CAD build for the part. Positions are in the model's coordinates, mm. A direction names the side the tool comes from. Give positions to 0.01 mm unless a question says otherwise; leave off trailing zeros. Answer as a JSON object with one key per item and string values.
```python
from build123d import *

# Parameters (mm, degrees)
CROQUIS1_R                          = 33
CROQUIS1_R_2                        = 29
BOSS_EXTRUDE1_DEPTH                 = 92
BOSS_EXTRUDE4_DEPTH                 = 15
SKETCH9_R                           = 1.75
CUT_EXTRUDE3_DEPTH                  = 14
SKETCH10_W                          = 7
SKETCH10_H                          = 15
SKETCH10_W_2                        = 8
SKETCH10_H_2                        = 13
CORTE_USB_Y_SWITCH_DEPTH            = 10
SKETCH11_W                          = 8
SKETCH11_H                          = 13
CUT_EXTRUDE5_DEPTH                  = 10
ALOJAMIENTO_TUERCA_DEPTH            = 2.2
ALOJAMIENTOS_TUERCAS_SUPERIOR_COUNT = 4
GROSOR_START                        = -47
SKETCH13_R                          = 29
SKETCH13_R_2                        = 26
GROSOR_ADICIONAL_DEPTH              = 47
CORTE_REVOLUCION_W                  = 30
CORTE_REVOLUCION_H                  = 8
CUT_REVOLVE3_ANGLE                  = 57
CIRPATTERN3_COUNT                   = 3
CORTE_POSTIZOS_DEPTH                = 44
CHAMFER3_SIZE                       = 3
SKETCH14_R                          = 1.75
CUT_EXTRUDE6_DEPTH                  = 17
TUERCAS_INFERIOR_DEPTH              = 2.2


with BuildPart() as part:
    # Croquis1 → Boss-Extrude1 (new body)
    with BuildSketch(Plane.XY):
        Circle(CROQUIS1_R)
        Circle(CROQUIS1_R_2, mode=Mode.SUBTRACT)
    extrude(amount=BOSS_EXTRUDE1_DEPTH)

    # Sketch8 → Boss-Extrude4 (add)
    with BuildSketch(Plane(origin=(0, 0, 0), x_dir=(-1, 0, 0), z_dir=(0, 0, -1))):
        with BuildLine():
            ThreePointArc((-4, -28.722813233), (0, -29), (4, -28.722813233))
            ThreePointArc((4, -28.722813233), (0, -26.000786616), (-4, -28.722813233))
        make_face()
        with BuildLine():
            ThreePointArc((-28.722813233, 4), (-29, 0), (-28.722813233, -4))
            ThreePointArc((-28.722813233, -4), (-26.000786616, 0), (-28.722813233, 4))
        make_face()
        with BuildLine():
            ThreePointArc((4, 28.722813233), (0, 29), (-4, 28.722813233))
            ThreePointArc((-4, 28.722813233), (0, 26.000786616), (4, 28.722813233))
        make_face()
        with BuildLine():
            ThreePointArc((28.722813233, -4), (29, 0), (28.722813233, 4))
            ThreePointArc((28.722813233, 4), (26.000786616, 0), (28.722813233, -4))
        make_face()
    extrude(amount=-BOSS_EXTRUDE4_DEPTH)

    # Sketch9 → Cut-Extrude3 (cut)
    with BuildSketch(Plane(origin=(0, 0, 0), x_dir=(-1, 0, 0), z_dir=(0, 0, -1))):
        with Locations((0, -29)):
            Circle(SKETCH9_R)
        with Locations((-29, 0)):
            Circle(SKETCH9_R)
        with Locations((0, 29)):
            Circle(SKETCH9_R)
        with Locations((29, 0)):
            Circle(SKETCH9_R)
    extrude(amount=-CUT_EXTRUDE3_DEPTH, mode=Mode.SUBTRACT)

    # Sketch10 → Corte USB y Switch (cut)
    with BuildSketch(Plane(origin=(-23.334523779, -23.334523779, 0), x_dir=(0, 0, -1), z_dir=(-0.7071067811865488, -0.7071067811865464, 0))):
        with Locations((-7, 0)):
            Rectangle(SKETCH10_W, SKETCH10_H)
        with Locations((-38, 0)):
            Rectangle(SKETCH10_W_2, SKETCH10_H_2)
    extrude(amount=-CORTE_USB_Y_SWITCH_DEPTH, mode=Mode.SUBTRACT)

    # Sketch11 → Cut-Extrude5 (cut)
    with BuildSketch(Plane(origin=(12.362017583, 30.597067201, 0), x_dir=(0, 0, -1), z_dir=(0.37460659341590646, 0.9271838545667896, 0))):
        with Locations((-26.9, -0.5)):
            Rectangle(SKETCH11_W, SKETCH11_H)
    extrude(amount=-CUT_EXTRUDE5_DEPTH, mode=Mode.SUBTRACT)

    # Tuerca → Alojamiento tuerca (cut)
    with BuildSketch(Plane(origin=(0, 0, 3), x_dir=(-1, 0, 0), z_dir=(0, 0, -1))):
        with BuildLine():
            Line((-29, -3.406366588), (-25.579878574, -3.406366588))
            ThreePointArc((-25.579878574, -3.406366588), (-23.904124497, 0), (-25.579878574, 3.406366588))
            Line((-25.579878574, 3.406366588), (-29, 3.406366588))
            Line((-29, 3.406366588), (-31.95, 1.703183294))
            Line((-31.95, 1.703183294), (-31.95, -1.703183294))
            Line((-31.95, -1.703183294), (-29, -3.406366588))
        make_face()
    alojamiento_tuerca = extrude(amount=-ALOJAMIENTO_TUERCA_DEPTH, mode=Mode.SUBTRACT)

    # Alojamientos Tuercas Superior: Alojamiento tuerca ×4 about axis
    alojamientos_tuercas_superior_axis = Axis((0, 0, 0), (0, 0, 1))
    for i in range(1, ALOJAMIENTOS_TUERCAS_SUPERIOR_COUNT):
        add(alojamiento_tuerca.rotate(alojamientos_tuercas_superior_axis, i * 360 / ALOJAMIENTOS_TUERCAS_SUPERIOR_COUNT), mode=Mode.SUBTRACT)

    # Sketch13 → Grosor adicional (add)
    with BuildSketch(Plane.XY.offset(92).offset(GROSOR_START)):
        with Locations(Location((0, 0, 0), (0, 0, 187.928141766))):
            Circle(SKETCH13_R)
        Circle(SKETCH13_R_2, mode=Mode.SUBTRACT)
    extrude(amount=GROSOR_ADICIONAL_DEPTH)

    # Corte Revolucion → Cut-Revolve3 (revolve, cut)
    with BuildSketch(Plane(origin=(0, 0, 0), x_dir=(0, 0, -1), z_dir=(0.2756373558169964, -0.9612616959383197, 0))):
        with Locations((-65, 29)):
            Rectangle(CORTE_REVOLUCION_W, CORTE_REVOLUCION_H)
    cut_revolve3 = revolve(axis=Axis((0, 0, 92), (0, 0, -1)), revolution_arc=CUT_REVOLVE3_ANGLE, mode=Mode.SUBTRACT)

    # CirPattern3: Cut-Revolve3 ×3 about axis
    cirpattern3_axis = Axis((0, 0, 0), (0, 0, 1))
    for i in range(1, CIRPATTERN3_COUNT):
        add(cut_revolve3.rotate(cirpattern3_axis, i * 360 / CIRPATTERN3_COUNT), mode=Mode.SUBTRACT)

    # Croquis2 → Corte postizos (cut)
    with BuildSketch(Plane.XY.offset(92)):
        with BuildLine():
            Line((7.72153797, 29.247911915), (7.338651789, 27.797602233))
            ThreePointArc((7.338651789, 27.797602233), (-8.645291736, 27.419362334), (-21.955521244, 18.561184955))
            Line((-21.955521244, 18.561184955), (-23.1010267, 19.529594604))
            ThreePointArc((-23.1010267, 19.529594604), (-9.096350435, 28.84993776), (7.72153797, 29.247911915))
        make_face()
        with BuildLine():
            Line((21.468665741, -21.311003996), (20.404103804, -20.254259996))
            ThreePointArc((20.404103804, -20.254259996), (28.068510205, -6.222638901), (27.052218317, 9.733446673))
            Line((27.052218317, 9.733446673), (28.463638403, 10.241278673))
            ThreePointArc((28.463638403, 10.241278673), (29.532954215, -6.547298322), (21.468665741, -21.311003996))
        make_face()
        with BuildLine():
            Line((-29.190203711, -7.936907919), (-27.742755593, -7.543342237))
            ThreePointArc((-27.742755593, -7.543342237), (-19.423218469, -21.196723433), (-5.096697073, -28.294631628))
            Line((-5.096697073, -28.294631628), (-5.362611703, -29.770873278))
            ThreePointArc((-5.362611703, -29.770873278), (-20.43660378, -22.302639439), (-29.190203711, -7.936907919))
        make_face()
    extrude(amount=-CORTE_POSTIZOS_DEPTH, mode=Mode.SUBTRACT)

    # Chamfer3
    chamfer3_edges = [part.edges().sort_by_distance(p)[0] for p in [
        (-29, 0, 45),
    ]]
    chamfer(chamfer3_edges, length=CHAMFER3_SIZE - 0.0001)  # a hair under: the kernel refuses the full size

    # Sketch14 → Cut-Extrude6 (cut)
    with BuildSketch(Plane.XY.offset(92)):
        with Locations((19.929911125, 21.749681436)):
            Circle(SKETCH14_R)
        with Locations((8.870821085, -28.134650047)):
            Circle(SKETCH14_R)
        with Locations((-28.80073221, 6.384968611)):
            Circle(SKETCH14_R)
    extrude(amount=-CUT_EXTRUDE6_DEPTH, mode=Mode.SUBTRACT)

    # Sketch15 → Tuercas inferior (cut)
    with BuildSketch(Plane.XY.offset(89)):
        with BuildLine():
            Line((17.415459305, 24.047694791), (15.108166619, 21.523089667))
            ThreePointArc((15.108166619, 21.523089667), (16.492116143, 17.98809762), (20.137070258, 16.927062957))
            Line((20.137070258, 16.927062957), (22.444362944, 19.451668081))
            Line((22.444362944, 19.451668081), (23.177274978, 22.778253911))
            Line((23.177274978, 22.778253911), (20.662823159, 25.076267266))
            Line((20.662823159, 25.076267266), (17.415459305, 24.047694791))
        make_face()
        with BuildLine():
            Line((12.118184939, -27.106077572), (11.08545911, -23.84560093))
            ThreePointArc((11.08545911, -23.84560093), (7.332091433, -23.276640352), (4.590731403, -25.90274588))
            Line((4.590731403, -25.90274588), (5.623457232, -29.163222522))
            Line((5.623457232, -29.163222522), (8.137909051, -31.461235877))
            Line((8.137909051, -31.461235877), (11.385272905, -30.432663402))
            Line((11.385272905, -30.432663402), (12.118184939, -27.106077572))
        make_face()
        with BuildLine():
            Line((-29.533644244, 3.058382781), (-26.193625729, 2.322511264))
            ThreePointArc((-26.193625729, 2.322511264), (-23.824207576, 5.288542732), (-24.727801661, 8.975682923))
            Line((-24.727801661, 8.975682923), (-28.067820176, 9.711554441))
            Line((-28.067820176, 9.711554441), (-31.31518403, 8.682981966))
            Line((-31.31518403, 8.682981966), (-32.048096064, 5.356396136))
            Line((-32.048096064, 5.356396136), (-29.533644244, 3.058382781))
        make_face()
    extrude(amount=-TUERCAS_INFERIOR_DEPTH, mode=Mode.SUBTRACT)


solid = part.part
```
1) Slice it at A-A (x = 0). State how many separate pieces and enclosed holes the cut face has, then the cut area to 3 significant figures.
Model answer:
{"separate pieces": "6", "enclosed holes": "0", "area": "777 mm2"}
2) Mould opens along Z. For faces 4 (the conical face through (-20.782, 15.935, 44.812)), 5 (the cylindrical face through (8.491, -29.843, 90.521)), 6 (the flat face through (-20, -23, 80)), 7 (the flat face through (0, 27, 0)) say: released by +Z, released by -Z, zero draft, split by the parting line, or undercut.
Model answer:
{"face 4": "undercut", "face 5": "zero draft", "face 6": "undercut", "face 7": "released by -Z"}
3) Wall check: probe 1 along Y at (x, z) = (0, 8); probe 2 along Z at (x, y) = (25, -18); probe 3 along Y at (x, z) = (-11.5, 87.5). Give the ranges that are in metal, low to high.
Model answer:
{"probe 1": "y = -33 to -30.75, -27.25 to -26, 26 to 27.25, 30.75 to 33", "probe 2": "z = 0 to 50, 80 to 92", "probe 3": "y = -30.93 to -27.98, -26.35 to -23.32, 23.32 to 26.35, 27.98 to 30.93"}
4) Pin check, flat tips, straight feed: pin 1 (3 mm diameter, centred on x = 22.5, z = 39, fed in from +Y); pin 2 (0.7 mm diameter, centred on x = 0.5, z = 4, fed in from -Y); pin 3 (4 mm diameter, centred on y = 4.5, z = 63, fed in from +X). Stop position of each tip, or through.
Model answer:
{"pin 1": "stops at y = 25.46", "pin 2": "stops at y = -33", "pin 3": "stops at x = -25.17"}
5) 3-axis set-ups, long thin cutter, end or side, ignore diameter. For faces 1 (the cylindrical face through (-12.845, 27.387, 84.975)), 2 (the flat face through (-26.047, -16.855, 38.056)), 3 (the flat face through (7, -27, 86.8)): which of +Z, -Z, +X, -X, +Y, -Y reach the whole face in a straight line?
Model answer:
{"face 1": "+Z", "face 2": "-Y", "face 3": "none"}
